Geometry check sheet. Reference: the model listing, model coordinates, mm. Face numbers are marked on the shaded views. A direction names the side the tool comes from. Coordinates: 2 decimals unless noted, no trailing zeros. Loops run counter-clockwise (first coordinate to the right, second up) from the corner with the lowest first, then second, coordinate; pieces in that order, holes last.
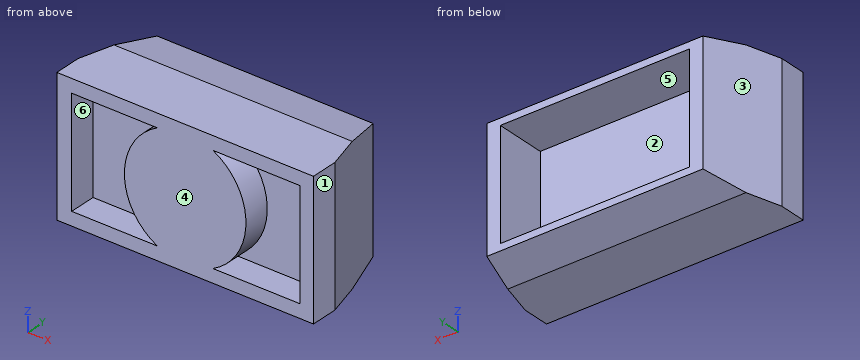
from build123d import *

# Parameters (mm, degrees)
SKETCH005_W      = 16.898421
SKETCH005_H      = 8
EXTRUDE004_DEPTH = 2.5
SKETCH_W         = 19
SKETCH_H         = 2
EXTRUDE_DEPTH    = 10
SKETCH012_R      = 4.5
EXTRUDE009_DEPTH = 2
EXTRUDE008_DEPTH = 19
SKETCH003_W      = 14
SKETCH003_H      = 8
EXTRUDE002_DEPTH = 3.75
EXTRUDE001_DEPTH = 10


with BuildPart() as extrude004:
    # Sketch005 (on Face2 of Extrude) → Extrude004 (new body, symmetric)
    with BuildSketch(Plane.XZ):
        with Locations((0.05079, 5)):
            Rectangle(SKETCH005_W, SKETCH005_H)
    extrude(amount=EXTRUDE004_DEPTH, both=True)


with BuildPart() as cut001:
    # Sketch → Extrude (new body)
    with BuildSketch(Plane.XY):
        with Locations((0, 1)):
            Rectangle(SKETCH_W, SKETCH_H)
    extrude(amount=EXTRUDE_DEPTH)

    # Cut001: cut Extrude004
    add(extrude004.part, mode=Mode.SUBTRACT)


with BuildPart() as extrude009:
    # Sketch012 (on Face7 of Common) → Extrude009 (new body)
    with BuildSketch(Plane.XZ.offset(-2)):
        with Locations((0, 5)):
            Circle(SKETCH012_R)
    extrude(amount=EXTRUDE009_DEPTH)


with BuildPart() as extrude008:
    # Sketch011 (on Face1 of Cut001) → Extrude008 (new body)
    with BuildSketch(Plane(origin=(-9.5, 0, 0), x_dir=(0, -1, 0), z_dir=(-1, 0, 0))):
        Polygon((-1.5, 10.5), (-7.5, 9.5), (-7.5, 0.5), (-1.5, -0.5), align=None)
    extrude(amount=-EXTRUDE008_DEPTH)


with BuildPart() as extrude002:
    # Sketch003 (on Face2 of Extrude001) → Extrude002 (new body, symmetric)
    with BuildSketch(Plane(origin=(0, 7.5, 0), x_dir=(-1, 0, 0), z_dir=(0, 1, 0))):
        with Locations((0, 5)):
            Rectangle(SKETCH003_W, SKETCH003_H)
    extrude(amount=EXTRUDE002_DEPTH, both=True)


with BuildPart() as fusion002:
    # Sketch001 → Extrude001 (new body)
    with BuildSketch(Plane.XY):
        Polygon((-9.5, 2), (-8, 7.5), (8, 7.5), (9.5, 2), align=None)
    extrude(amount=EXTRUDE001_DEPTH)

    # Cut: cut Extrude002
    add(extrude002.part, mode=Mode.SUBTRACT)

    # Common: intersect Extrude008
    add(extrude008.part, mode=Mode.INTERSECT)

    # Fusion001: union Extrude009
    add(extrude009.part)

    # Fusion002: union Cut001
    add(cut001.part)


solid = fusion002.part
1) Material ranges on probe 1 along Z at (x, y) = (5.5, 1); probe 2 along Y at (x, z) = (-2.75, 7.75); probe 3 along Y at (x, z) = (-4.5, 6), recorded low to high.
Data:
probe 1: z = 0 to 1, 9 to 10
probe 2: y = 0 to 3.75
probe 3: y = 2 to 3.75
2) Section check B-B on x = 1.5. Record the cut outline in (y, z).
Data:
outline: (0, 0) - (4.5, 0) - (7.5, 0.5) - (7.5, 1) - (3.75, 1) - (3.75, 9) - (7.5, 9) - (7.5, 9.5) - (4.5, 10) - (0, 10) - close
3) Section check A-A on y = 1. Record the cut outline in (x, z).
Data:
outline: (-9.5, 0) - (9.5, 0) - (9.5, 10) - (-9.5, 10) - close; hole (-8.4, 1) - (-2.06, 1) arc R4.5 cw to (-2.06, 9) - (-8.4, 9) - close; hole (2.06, 1) - (8.5, 1) - (8.5, 9) - (2.06, 9) arc R4.5 cw to start
4) Depth check by flat-ended pin: pin 1 (3 mm diameter, centred on y = 5.5, z = 6.5, fed in from +X); pin 2 (1.6 mm diameter, centred on x = -5, y = 1.5, fed in from -Z); pin 3 (2 mm diameter, centred on y = 4, z = 9, fed in from -X); pin 4 (1.9 mm diameter, centred on x = -2, y = 6, fed in from +Z). Enter the tip coordinate at first touch or a pass-through.
Data:
pin 1: stops at x = 8.95
pin 2: stops at z = 0
pin 3: stops at x = -9.23
pin 4: stops at z = 9.91
5) Section check C-C on y = 6. Record the cut outline in (x, z).
Data:
outline: (-8.41, 0.25) - (8.41, 0.25) - (8.41, 9.75) - (-8.41, 9.75) - close; hole (-7, 1) - (7, 1) - (7, 9) - (-7, 9) - close
6) Access from +Z, -Z, +X, -X, +Y, -Y to the whole of each face (thin tool, end or side, straight path). Record for the marked faces 4, 5 and 6.
Data:
face 4: +Z, -Z, +X, -X, -Y
face 5: +Y
face 6: -Y
7) Mould release check, pull along X, two halves, no side actions. Record for the marked faces 1, 2 and 3: +X half, -X half, draft (parallel to the pull), parting line (faces both ways), or undercut.
Data:
face 1: +X half
face 2: undercut
face 3: -X half
8) Section check D-D on z = 7.25. Record the cut outline in (x, y).
Data:
outline: (-9.5, 0) - (-8.4, 0) - (-8.4, 2) - (-3.9, 2) - (-3.9, 0) - (3.9, 0) - (3.9, 2) - (8.5, 2) - (8.5, 0) - (9.5, 0) - (9.5, 2) - (8, 7.5) - (7, 7.5) - (7, 3.75) - (-7, 3.75) - (-7, 7.5) - (-8, 7.5) - (-9.5, 2) - close
